CAD build for the part. Positions are in the model's coordinates, mm. A direction names the side the tool comes from. Coordinates: 2 decimals unless noted, no trailing zeros. Loops run counter-clockwise (first coordinate to the right, second up) from the corner with the lowest first, then second, coordinate; pieces in that order, holes last. Notation, with made-up numbers: (72, -12) -> (119, -12) arc R9 ccw to (119, 2) -> close; hole circle Ø7 at (35.25, 40). An arc over 180 degrees is marked (long way). Answer as a JSON object with one key per item and string values. Group by question number.
from build123d import *

# Parameters (mm, degrees)
BOSS_EXTRUDE1_DEPTH      = 150
BOSS_EXTRUDE1_DEPTH_BACK = 150
SKETCH3_W                = 50
SKETCH3_H                = 125
BOSS_EXTRUDE2_DEPTH      = 125
SKETCH4_W                = 100
SKETCH4_H                = 125
CUT_EXTRUDE1_DEPTH       = 230


with BuildPart() as part:
    # Sketch1 → Boss-Extrude1 (new, two sides: drawn at the far end of the back side and taken through both)
    with BuildSketch(Plane(origin=(0, 0, 0), x_dir=(0, 0, -1), z_dir=(1, 0, 0)).offset(-BOSS_EXTRUDE1_DEPTH_BACK)):
        Polygon((0, 0), (-175, 0), (-175, 25), (-150, 25), (-150, 75), (-350, 75), (-350, 25), (-325, 25), (-325, 0), (-500, 0), (-500, 325), (-375, 200), (-150, 200), (0, 325), align=None)
    extrude(amount=BOSS_EXTRUDE1_DEPTH + BOSS_EXTRUDE1_DEPTH_BACK)

    # Sketch3 → Boss-Extrude2 (add)
    with BuildSketch(Plane(origin=(0, 200, 0), x_dir=(1, 0, 0), z_dir=(0, 1, 0))):
        with Locations((125, -437.5)):
            Rectangle(SKETCH3_W, SKETCH3_H)
        with Locations((-125, -437.5)):
            Rectangle(SKETCH3_W, SKETCH3_H)
    extrude(amount=BOSS_EXTRUDE2_DEPTH)

    # Sketch4 → Cut-Extrude1 (cut)
    with BuildSketch(Plane(origin=(0, 0, 0), x_dir=(-1, 0, 0), z_dir=(0, 0, -1))):
        with Locations((0, 262.5)):
            Rectangle(SKETCH4_W, SKETCH4_H)
    extrude(amount=-CUT_EXTRUDE1_DEPTH, mode=Mode.SUBTRACT)


solid = part.part
Item 1: Band-saw the part on A-A, the plane y = 242. List the corners of the cut face in (x, z).
Item 2: Band-saw the part on D-D, the plane z = 109.5. List the corners of the cut face in (x, y), and give its area (4 significant figures).
Item 3: 3-axis set-ups, long thin cutter, end or side, ignore diameter. For faces 1 (the flat face through (125, 262, 375)), 2 (the flat face through (-1, 263, 438)), 3 (the flat face through (-2, 75, 249)), 4 (the flat face through (-2, 13, 325)), 5 (the flat face through (50, 248, 57)): which of +Z, -Z, +X, -X, +Y, -Y reach the whole face in a straight line?
Item 4: Band-saw the part on B-B, the plane y = 57.5. List the corners of the cut face in (x, z).
Item 5: Band-saw the part on C-C, the plane x = 71.5. List the corners of the cut face in (y, z).
Item 6: Pull direction Z, two halves, no side cores. Call faces 6 (the flat face through (-2, 0, 86)), 7 (the flat face through (-100.7, 261.625, 76.05)), 8 (the flat face through (-2, 160, 500)): +Z half, -Z half, draft (parallel to the pull), parting line (faces both ways), or undercut.
Item 7: Drill centre lines: L1, parallel to Z at x = 96.5, y = 36; L2, parallel to X at y = 260.5, z = 426; L3, parallel to Y at x = 103, z = 225. Where is each one in solid material? Low to high.
Item 8: Flat gauge pins, fed straight in: P1, Ø1, axis at x = 69.5, z = 278.5, coming from the -Y side; P2, Ø7.5, axis at x = -50, z = 161, coming from the +Y side. Where does each tip first touch, or does it go through?
Reply:
{
 "1": {"outline": "(-150, 0) -> (-50, 0) -> (-50, 99.6) -> (-150, 99.6) -> close; (-150, 375) -> (-100, 375) -> (-100, 417) -> (100, 417) -> (100, 375) -> (150, 375) -> (150, 500) -> (-150, 500) -> close; (50, 0) -> (150, 0) -> (150, 99.6) -> (50, 99.6) -> close"},
 "2": {"outline": "(-150, 0) -> (150, 0) -> (150, 233.75) -> (50, 233.75) -> (50, 200) -> (-50, 200) -> (-50, 233.75) -> (-150, 233.75) -> close", "area": "66,750 mm²"},
 "3": {"face 1": "+X, -X, +Y", "face 2": "+Y", "face 3": "+X, -X", "face 4": "+X, -X, -Y", "face 5": "-Z, +Y"},
 "4": {"outline": "(-150, 0) -> (150, 0) -> (150, 150) -> (-150, 150) -> close; (-150, 350) -> (150, 350) -> (150, 500) -> (-150, 500) -> close"},
 "5": {"outline": "(0, 0) -> (325, 0) -> (200, 150) -> (200, 375) -> (325, 500) -> (0, 500) -> (0, 325) -> (25, 325) -> (25, 350) -> (75, 350) -> (75, 150) -> (25, 150) -> (25, 175) -> (0, 175) -> close"},
 "6": {"face 6": "draft", "face 7": "undercut", "face 8": "+Z half"},
 "7": {"L1": "0 to 150, 350 to 500", "L2": "-150 to -100, 100 to 150", "L3": "75 to 200"},
 "8": {"P1": "y = 75", "P2": "y = 200"}
}
